Geometry check sheet. Reference: the model listing, model coordinates, mm. A direction names the side the tool comes from. Give positions to 0.01 mm unless a question says otherwise; leave off trailing zeros. Write each loop counter-clockwise with the first axis right and the second up, starting at its lowest first coordinate (ties: lowest second). Pieces come first, ordered by that corner, then holes. Notation, with made-up numbers: M 61,55 L 97,55 A30 cw 97,92 Z; hole C 87.5,79 d9. An arc over 180 degrees is marked long. Write each question's results on one line, items separated by ' | '.
```python
from build123d import *

# Parameters (mm, degrees)
SKETCH_1_R      = 2
SKETCH_1_R_2    = 1.5
SKETCH_1_R_3    = 1
EXTRUDE_1_DEPTH = 3
FILLET_1_R      = 1


with BuildPart() as part:
    # 草图1 → 凸台-拉伸1 (new body)
    with BuildSketch(Plane.XY):
        with BuildLine():
            Line((0, 7.5), (5, 7.5))
            Line((5, 7.5), (5, 10.5))
            Line((5, 10.5), (15, 10.5))
            Line((15, 10.5), (15, 7.5))
            Line((15, 7.5), (35, 7.5))
            Line((35, 7.5), (35, 10.5))
            Line((35, 10.5), (45, 10.5))
            Line((45, 10.5), (45, 7.5))
            Line((45, 7.5), (54.330127019, 7.5))
            ThreePointArc((54.330127019, 7.5), (55.624222244, 7.670370869), (56.830127019, 8.169872981))
            Line((56.830127019, 8.169872981), (66, 13.464101615))
            ThreePointArc((66, 13.464101615), (70.828427125, 12.828427125), (71.464101615, 8))
            Line((71.464101615, 8), (68.134857418, 2.2335799))
            ThreePointArc((68.134857418, 2.2335799), (67.182681437, 1.047193216), (65.917821708, 0.202040965))
            Line((65.917821708, 0.202040965), (50.405359552, -7.031538935))
            ThreePointArc((50.405359552, -7.031538935), (49.374466313, -7.381480036), (48.292268243, -7.5))
            Line((48.292268243, -7.5), (45, -7.5))
            Line((45, -7.5), (45, -10.5))
            Line((45, -10.5), (35, -10.5))
            Line((35, -10.5), (35, -7.5))
            Line((35, -7.5), (15, -7.5))
            Line((15, -7.5), (15, -10.5))
            Line((15, -10.5), (5, -10.5))
            Line((5, -10.5), (5, -7.5))
            Line((5, -7.5), (0, -7.5))
            Line((0, -7.5), (0, 7.5))
        make_face()
        with Locations((68, 10)):
            Circle(SKETCH_1_R, mode=Mode.SUBTRACT)
        with Locations((5, 0)):
            Circle(SKETCH_1_R_2, mode=Mode.SUBTRACT)
        with Locations((45, 0)):
            Circle(SKETCH_1_R_2, mode=Mode.SUBTRACT)
        with Locations((18, 0)):
            Circle(SKETCH_1_R, mode=Mode.SUBTRACT)
        with Locations((62, 9)):
            Circle(SKETCH_1_R_3, mode=Mode.SUBTRACT)
    extrude(amount=EXTRUDE_1_DEPTH)

    # 圆角1
    fillet_1_edges = [part.edges().sort_by_distance(p)[0] for p in [
        (0, 7.5, 1.5),
        (5, 10.5, 1.5),
        (15, 10.5, 1.5),
        (35, 10.5, 1.5),
        (45, 10.5, 1.5),
        (45, -10.5, 1.5),
        (35, -10.5, 1.5),
        (15, -10.5, 1.5),
        (5, -10.5, 1.5),
        (0, -7.5, 1.5),
    ]]
    fillet(fillet_1_edges, radius=FILLET_1_R)


solid = part.part
```
Q1. Section check D-D (x = 39). Enter the section's corners in (y, z), then the cut area to 3 significant figures.
Answer key:
outline: M -10.5,0 L 10.5,0 L 10.5,3 L -10.5,3 Z | area: 63.0 mm2
Q2. Section check A-A (y = 11.25). Enter the section's corners in (x, z).
Answer key:
outline: M 62.17,0 L 66.44,0 L 66.44,3 L 62.17,3 Z; M 69.56,0 L 71.8,0 L 71.8,3 L 69.56,3 Z
Q3. Material ranges on probe 1 along Y at (x, z) = (68, 1.05); probe 2 along Y at (x, z) = (18, 0.6); probe 3 along X at (y, z) = (0.25, 2), recorded low to high. Write a range as [from, to].
Answer key:
probe 1: y = [2.01, 8], [12, 14] | probe 2: y = [-7.5, -2], [2, 7.5] | probe 3: x = [0, 3.52], [6.48, 16.02], [19.98, 43.52], [46.48, 66.02]
Q4. Depth check by flat-ended pin: P1, Ø1, axis at y = 8.5, z = 2, coming from the +X side; P2, Ø1.5, axis at x = 2.5, z = 1, coming from the +Y side; P3, Ø1.6, axis at y = 9, z = 2, coming from the -X side. Enter the tip coordinate at first touch or a pass-through.
Answer key:
P1: stops at x = 71.87 | P2: stops at y = 7.5 | P3: stops at x = 5
Q5. Section check C-C (z = 1.4). State how many separate pieces and enclosed holes the cut face has, then the cut area to 3 significant figures.
Answer key:
separate pieces: 1 | enclosed holes: 5 | area: 1,090 mm2
Q6. Section check B-B (x = 19). Enter the section's corners in (y, z), then the cut area to 3 significant figures.
Answer key:
outline: M -7.5,0 L -1.73,0 L -1.73,3 L -7.5,3 Z; M 1.73,0 L 7.5,0 L 7.5,3 L 1.73,3 Z | area: 34.6 mm2
Q7. Release check for a two-part mould opening along Y. For faces 1 (the face through (61, 9, 1)), 2 (the face through (35, 8, 1)), 3 (the face through (58.27, -3.364, 1.479)) record: released by +Y, released by -Y, zero draft, split by the parting line, or undercut.
Answer key:
face 1: undercut | face 2: zero draft | face 3: released by -Y
Q8. Access from +Z, -Z, +X, -X, +Y, -Y to the whole of each face (thin tool, end or side, straight path). Record for faces 4 (the face through (35, -9, 1)), 5 (the face through (45, 9, 1)), 6 (the face through (47, -7.5, 1)), 7 (the face through (3, 7.5, 1)), 8 (the face through (5, -9, 1)).
Answer key:
face 4: +Z, -Z, -Y | face 5: +Z, -Z, +Y | face 6: +Z, -Z, +X, -Y | face 7: +Z, -Z, -X, +Y | face 8: +Z, -Z, -X, -Y
